Autodesk Fusion 360 part; units mm, degrees
sketch "Boceto1" plane through (0, 0, 0) normal (0, 0, 1) x (1, 0, 0)
  circle A0 centre (0, 0) radius 14.45
  circle A1 centre (0, 0) radius 17.125
  circle A2 centre (0, 0) radius 4
  circle A3 centre (0, 0) radius 5
  circle A4 centre (0, 0) radius 8
  line L0 (0, 0) -> (0, 11.225)
  circle A5 centre (0, 11.225) radius 1.5
  circle A6 centre (-11.225, 0) radius 1.5
  circle A7 centre (0, -11.225) radius 1.5
  circle A8 centre (11.225, 0) radius 1.5
  dimension "d1" = 28.9
  dimension "d2" = 34.25
  dimension "d7" = 8
  dimension "d8" = 10
  dimension "d13" = 16
  dimension "d22" = 11.225
  dimension "d23" = 3
  dimension "d25" = 360
extrude "Extruir1" add sketch "Boceto1" along normal blind 80.4 contours A0 | A2 | A3 | A4 | A5 | A6 | A7 | A8
extrude "Extruir2" add sketch "Boceto1" along normal blind 42.6 contours A1
extrude "Extruir3" add sketch "Boceto1" along normal blind 83.6 contours A2 | A3
extrude "Extruir4" add sketch "Boceto1" against normal blind 27 contours A2
extrude "Extruir5" add sketch "Boceto1" against normal blind 1.7 contours A4
sketch "Boceto2" plane through (0, 0, 0) normal (0, 1, 0) x (1, 0, 0)
  line L0 (4, 27) -> (4, 2.5)
  line L1 (-4, 2.5) -> (-4, 27)
  line L2 (4, 27) -> (-4, 27)
  line L3 (4, 27) -> (-4, 27)
  line L4 (-4, 0) -> (4, 0)
  line L5 (4, 27) -> (-4, 27)
  line L6 (0, 27) -> (0, 16.1)
  line L7 (0, 16.1) -> (0, 14.1)
  circle A0 centre (0, 14.1) radius 2
  dimension "d26" = 10.9
  dimension "d27" = 2
  dimension "d28" = 4
extrude "Extruir7" cut sketch "Boceto2" along normal mid plane 14
Check sheet for the modelled part. Datum: model origin and axes. Units: mm. A direction names the side the tool comes from. Round coordinates to 2 decimals unless told otherwise and drop trailing zeros. Order: outer loops, then holes, each group sorted by start corner. A loop starts at its lowest first (then second) coordinate and runs counter-clockwise, first axis right, second up. Notation, with made-up numbers: M 44,50.25 L 53,50.25 A16 ccw 53,78.25 Z; hole C 15,82.25 d2. An arc over 180 degrees is marked long. One line per item, written item: value. Start each with the question number.
1. Section check C-C on z = -6.5. Enter the section's corners in (x, y), and give its area (3 significant figures).
2. Section check A-A on x = 0. Enter the section's corners in (y, z) (3 decimals), and give its area (3 significant figures).
3. Gauge pin test, flat ends, axial feed: P1, Ø1.5, axis at y = -7, z = 63, coming from the -X side; P2, Ø5, axis at y = -8.5, z = 29.5, coming from the +X side; P3, Ø6, axis at x = -6.5, z = -9, coming from the +Y side. Record the tip position at first contact, or that the pin passes through.
4. Release check for a two-part mould opening along X. For faces 4 (the cylindrical face through (16.334, -5.144, 21.002)), 5 (the flat face through (0, -6, 80.4)), 6 (the cylindrical face through (1.847, -0.056, -14.866)) record: released by +X, released by -X, zero draft, split by the parting line, or undercut.
5. Section check B-B on y = 0. Enter the section's corners in (x, z) (3 decimals), and give its area (3 significant figures).
6. Section check D-D on x = -10.5. Enter the section's corners in (y, z).
7. Scan lines: line 1 along Y through (x, z) = (0, -1); line 2 along Z through (x, y) = (0, 1); line 3 along Z through (x, y) = (-4, 1.5). Record each from-to range of solid material in increasing order.
8. Access from +Z, -Z, +X, -X, +Y, -Y to the whole of each face (thin tool, end or side, straight path). Record for faces 1 (the flat face through (-8, -13, 42.6)), 2 (the flat face through (-0.1, -5.2, -1.7)), 3 (the flat face through (0, 0, 83.6)).
Results found:
1. outline: C 0,0 d8
1. area: 50.3 mm^2
2. outline: M -17.125,0 L -8,0 L -8,-1.7 L -5,-1.7 L -5,0 L -4,0 L -4,-12.1 L 4,-12.1 L 4,0 L 5,0 L 5,-1.7 L 8,-1.7 L 8,0 L 17.125,0 L 17.125,42.6 L 14.45,42.6 L 14.45,80.4 L 5,80.4 L 5,83.6 L -5,83.6 L -5,80.4 L -14.45,80.4 L -14.45,42.6 L -17.125,42.6 Z; M -4,-27 L 4,-27 L 4,-16.1 L -4,-16.1 Z
2. area: 2,780 mm^2
3. P1: x = -13.03
3. P2: x = 16.04
3. P3: y = 1.94
4. face 4: split by the parting line
4. face 5: zero draft
4. face 6: undercut
5. outline: M -17.125,0 L -8,0 L -8,-1.7 L -5,-1.7 L -5,0 L -4,0 L -4,-27 L 4,-27 L 4,0 L 5,0 L 5,-1.7 L 8,-1.7 L 8,0 L 17.125,0 L 17.125,42.6 L 14.45,42.6 L 14.45,80.4 L 5,80.4 L 5,83.6 L -5,83.6 L -5,80.4 L -14.45,80.4 L -14.45,42.6 L -17.125,42.6 Z; hole C 0,-14.1 d4
5. area: 2,800 mm^2
6. outline: M -13.53,0 L 13.53,0 L 13.53,42.6 L 9.93,42.6 L 9.93,80.4 L -9.93,80.4 L -9.93,42.6 L -13.53,42.6 Z
7. line 1: -8 to -5, -4 to 4, 5 to 8
7. line 2: -27 to -16.1, -12.1 to 83.6
7. line 3: 0 to 83.6
8. face 1: +Z
8. face 2: -Z
8. face 3: +Z, +X, -X, +Y, -Y
